```python
from build123d import *

# Parameters (mm, degrees)
SKETCH1_W                = 100
SKETCH1_H                = 64
BOSS_EXTRUDE1_DEPTH      = 3
SKETCH2_W                = 100
SKETCH2_H                = 64
SKETCH2_W_2              = 96
SKETCH2_H_2              = 60
BOSS_EXTRUDE2_DEPTH      = 35
BOSS_EXTRUDE9_DEPTH      = 5
BOSS_EXTRUDE9_DEPTH_BACK = 37
SKETCH12_W               = 5
SKETCH12_H               = 5
CUT_EXTRUDE6_DEPTH       = 72.582120673
BOSS_EXTRUDE11_DEPTH     = 10
SKETCH19_W               = 5
SKETCH19_H               = 5
CUT_EXTRUDE7_DEPTH       = 7
FILLET2_R                = 10


with BuildPart() as part:
    # Sketch1 → Boss-Extrude1 (new body)
    with BuildSketch(Plane(origin=(0, 0, 0), x_dir=(1, 0, 0), z_dir=(0, 1, 0))):
        Rectangle(SKETCH1_W, SKETCH1_H)
    extrude(amount=BOSS_EXTRUDE1_DEPTH)

    # Sketch2 → Boss-Extrude2 (add)
    with BuildSketch(Plane(origin=(0, 3, 0), x_dir=(1, 0, 0), z_dir=(0, 1, 0))):
        Rectangle(SKETCH2_W, SKETCH2_H)
        Rectangle(SKETCH2_W_2, SKETCH2_H_2, mode=Mode.SUBTRACT)
    extrude(amount=BOSS_EXTRUDE2_DEPTH)

    # Sketch12 → Boss-Extrude9 (add, two sides: drawn at the far end of the back side and taken through both)
    with BuildSketch(Plane(origin=(0, 38, 0), x_dir=(1, 0, 0), z_dir=(0, 1, 0)).offset(-BOSS_EXTRUDE9_DEPTH_BACK)):
        with Locations((-45.5, 27.5)):
            Rectangle(SKETCH12_W, SKETCH12_H)
        with Locations((45.5, 27.5)):
            Rectangle(SKETCH12_W, SKETCH12_H)
        with Locations((45.5, -27.5)):
            Rectangle(SKETCH12_W, SKETCH12_H)
        with Locations((-45.5, -27.5)):
            Rectangle(SKETCH12_W, SKETCH12_H)
    extrude(amount=BOSS_EXTRUDE9_DEPTH + BOSS_EXTRUDE9_DEPTH_BACK)

    # Sketch14 → Cut-Extrude6 (cut, through all)
    with BuildSketch(Plane(origin=(0, 3, 0), x_dir=(1, 0, 0), z_dir=(0, 1, 0))):
        with BuildLine():
            Line((-46, -10), (-46, 10))
            ThreePointArc((-46, 10), (-41, 15), (-36, 10))
            Line((-36, 10), (-36, -10))
            ThreePointArc((-36, -10), (-41, -15), (-46, -10))
        make_face()
    extrude(amount=-CUT_EXTRUDE6_DEPTH, mode=Mode.SUBTRACT)

    # Sketch17 → Boss-Extrude11 (add)
    with BuildSketch(Plane(origin=(0, 3, 0), x_dir=(1, 0, 0), z_dir=(0, 1, 0))):
        Polygon((-38, 30), (-43, 30), (-43, 25), (-48, 25), (-48, 20), (-38, 20), align=None)
        Polygon((43, 30), (38, 30), (38, 20), (48, 20), (48, 25), (43, 25), align=None)
        Polygon((48, -25), (48, -20), (38, -20), (38, -30), (43, -30), (43, -25), align=None)
        Polygon((-38, -20), (-48, -20), (-48, -25), (-43, -25), (-43, -30), (-38, -30), align=None)
    extrude(amount=BOSS_EXTRUDE11_DEPTH)

    # Sketch19 → Cut-Extrude7 (cut)
    with BuildSketch(Plane.XZ):
        with Locations((-45.5, 27.5)):
            Rectangle(SKETCH19_W, SKETCH19_H)
        with Locations((45.5, 27.5)):
            Rectangle(SKETCH19_W, SKETCH19_H)
        with Locations((45.5, -27.5)):
            Rectangle(SKETCH19_W, SKETCH19_H)
        with Locations((-45.5, -27.5)):
            Rectangle(SKETCH19_W, SKETCH19_H)
    extrude(amount=-CUT_EXTRUDE7_DEPTH, mode=Mode.SUBTRACT)

    # Fillet2
    fillet2_edges = [part.edges().sort_by_distance(p)[0] for p in [
        (-38, 8, 20),
        (38, 8, -20),
        (38, 8, 20),
        (-38, 8, -20),
    ]]
    fillet(fillet2_edges, radius=FILLET2_R - 0.0001)  # a hair under: the kernel refuses the full size


solid = part.part
```
The model under review builds one solid part; all positions refer to its coordinate system, in mm. A direction names the side the tool comes from. Coordinates: 2 decimals unless noted, no trailing zeros. Write each loop counter-clockwise with the first axis right and the second up, starting at its lowest first coordinate (ties: lowest second). Pieces come first, ordered by that corner, then holes. Notation, with made-up numbers: (84, 56.5) - (100, 56.5) arc R27 cw to (100, 72.5) - close; hole circle Ø2 at (73.5, 86). An arc over 180 degrees is marked (long way). Answer in a Markdown table with one row per item. Add a question column.
Q1. Draft analysis for pull direction Z (two halves, no side actions). For faces 5 (the face through (-1, 19, 32)), 6 (the face through (45, 43, 27)), 7 (the face through (48, 3, 27)), state which applies: +Z half, -Z half, draft (parallel to the pull), parting line (faces both ways), or undercut.
Q2. Consider section D-D on x = -41. Give the boundary of the cut face in (y, z), then the cut area to 3 significant figures.
Q3. For faces 1 (the face through (45, 40, 30)), 2 (the face through (-48, 40, 28)), 3 (the face through (-46, 3, -25)), 4 (the face through (-48, 20, 0)), list the 3-axis set-ups (+Z, -Z, +X, -X, +Y, -Y) from which the entire face can be reached by the end or side of a thin tool; tool diameter is ignored.
Q4. Consider section C-C on z = 18. Give the boundary of the cut face in (x, y), then the cut area to 3 significant figures.
Q5. To check wall thickness, follow line 1 along Z through (x, y) = (-13, 23); line 2 along X through (y, z) = (18.5, -17); line 3 along Y through (x, z) = (-6.5, -23). State the ranges of each line that lie inside material, in increasing order. Write a range as from..to.
Q6. Clearance check with flat-ended pins moving along their axes: pin 1 (1.5 mm diameter, centred on x = 45.5, y = 41, fed in from +Z); pin 2 (1.5 mm diameter, centred on x = -45, z = -28, fed in from -Y); pin 3 (8 mm diameter, centred on x = -35, z = 18.5, fed in from +Y). State where each tip first meets the part, or that it passes through.
Q7. Consider section A-A on y = 29. Give the boundary of the cut face in (x, z).
Q8. Consider section B-B on x = 15. Give the boundary of the cut face in (y, z), then the cut area to 3 significant figures.
Answers below:
| question | item | result |
|---|---|---|
| 1 | face 5 | +Z half |
| 1 | face 6 | draft |
| 1 | face 7 | undercut |
| 2 | outline | (0, -32) - (38, -32) - (38, -30) - (13, -30) - (13, -22.86) - (3, -22.86) - (3, -15) - (0, -15) - close; (0, 15) - (3, 15) - (3, 22.86) - (13, 22.86) - (13, 30) - (38, 30) - (38, 32) - (0, 32) - close |
| 2 | area | 385 mm² |
| 3 | face 1 | +Z, +X, -X, +Y |
| 3 | face 2 | +Z, -Z, -X, +Y |
| 3 | face 3 | -Y |
| 3 | face 4 | +Y |
| 4 | outline | (-50, 0) - (50, 0) - (50, 38) - (48, 38) - (48, 3) - (-48, 3) - (-48, 38) - (-50, 38) - close |
| 4 | area | 440 mm² |
| 5 | line 1 | -32..-30, 30..32 |
| 5 | line 2 | -50..-48, 48..50 |
| 5 | line 3 | 0..3 |
| 6 | pin 1 | z = 30 |
| 6 | pin 2 | y = 7 |
| 6 | pin 3 | y = 3 |
| 7 | outline | (-50, -32) - (50, -32) - (50, 32) - (-50, 32) - close; hole (-48, -25) - (-43, -25) - (-43, -30) - (43, -30) - (43, -25) - (48, -25) - (48, 25) - (43, 25) - (43, 30) - (-43, 30) - (-43, 25) - (-48, 25) - close |
| 8 | outline | (0, -32) - (38, -32) - (38, -30) - (3, -30) - (3, 30) - (38, 30) - (38, 32) - (0, 32) - close |
| 8 | area | 332 mm² |
